```python
from build123d import *

# Parameters (mm, degrees)
SKETCH1_W           = 160
SKETCH1_H           = 50
BOSS_EXTRUDE1_DEPTH = 1.25
SKETCH2_W           = 10
SKETCH2_H           = 2.5
SKETCH2_W_2         = 15
CUT_EXTRUDE1_DEPTH  = 4
SKETCH3_W           = 2.5
SKETCH3_H           = 22.5
CUT_EXTRUDE2_DEPTH  = 84.852549156
CUT_EXTRUDE4_REACH  = 85.853
SKETCH4_R           = 5.5
SKETCH4_R_2         = 2.5


with BuildPart() as part:
    # Sketch1 → Boss-Extrude1 (new, symmetric)
    with BuildSketch(Plane(origin=(0, 0, 0), x_dir=(1, 0, 0), z_dir=(0, 1, 0))):
        Rectangle(SKETCH1_W, SKETCH1_H)
    extrude(amount=BOSS_EXTRUDE1_DEPTH, both=True)

    # Sketch2 → Cut-Extrude1 (cut)
    with BuildSketch(Plane(origin=(0, 1.25, 0), x_dir=(1, 0, 0), z_dir=(0, 1, 0))):
        with Locations((30, 23.75)):
            Rectangle(SKETCH2_W, SKETCH2_H)
        with Locations((10, 23.75)):
            Rectangle(SKETCH2_W, SKETCH2_H)
        with Locations((10, -23.75)):
            Rectangle(SKETCH2_W, SKETCH2_H)
        with Locations((30, -23.75)):
            Rectangle(SKETCH2_W, SKETCH2_H)
        with Locations((50, 23.75)):
            Rectangle(SKETCH2_W, SKETCH2_H)
        with Locations((50, -23.75)):
            Rectangle(SKETCH2_W, SKETCH2_H)
        with Locations((-10, 23.75)):
            Rectangle(SKETCH2_W, SKETCH2_H)
        with Locations((-10, -23.75)):
            Rectangle(SKETCH2_W, SKETCH2_H)
        with Locations((-30, 23.75)):
            Rectangle(SKETCH2_W, SKETCH2_H)
        with Locations((-30, -23.75)):
            Rectangle(SKETCH2_W, SKETCH2_H)
        with Locations((-50, 23.75)):
            Rectangle(SKETCH2_W, SKETCH2_H)
        with Locations((-50, -23.75)):
            Rectangle(SKETCH2_W, SKETCH2_H)
        with Locations((72.5, 23.75)):
            Rectangle(SKETCH2_W_2, SKETCH2_H)
        with Locations((72.5, -23.75)):
            Rectangle(SKETCH2_W_2, SKETCH2_H)
        with Locations((-72.5, 23.75)):
            Rectangle(SKETCH2_W_2, SKETCH2_H)
        with Locations((-72.5, -23.75)):
            Rectangle(SKETCH2_W_2, SKETCH2_H)
    extrude(amount=-CUT_EXTRUDE1_DEPTH, mode=Mode.SUBTRACT)

    # Sketch3 → Cut-Extrude2 (cut, through all)
    with BuildSketch(Plane(origin=(0, 1.25, 0), x_dir=(1, 0, 0), z_dir=(0, 1, 0))):
        with Locations((78.75, -11.25)):
            Rectangle(SKETCH3_W, SKETCH3_H)
        with Locations((-78.75, -11.25)):
            Rectangle(SKETCH3_W, SKETCH3_H)
    extrude(amount=-CUT_EXTRUDE2_DEPTH, mode=Mode.SUBTRACT)

    # Sketch4 → Cut-Extrude4 (cut, up to next)
    with BuildSketch(Plane.XZ.offset(1.25), mode=Mode.PRIVATE) as cut_extrude4_sk1:
        with Locations(Location((-57.7529076, -6.3187203, 0), (0, 0, 270))):
            Circle(SKETCH4_R)
    cut_extrude4_tool1 = extrude(cut_extrude4_sk1.sketch, amount=-CUT_EXTRUDE4_REACH, mode=Mode.PRIVATE) & part.part
    # Sketch4 → Cut-Extrude4 (cut, up to next)
    with BuildSketch(Plane.XZ.offset(1.25), mode=Mode.PRIVATE) as cut_extrude4_sk2:
        with Locations(Location((-27.7529076, 0, 0), (0, 0, 270))):
            Circle(SKETCH4_R_2)
    cut_extrude4_tool2 = extrude(cut_extrude4_sk2.sketch, amount=-CUT_EXTRUDE4_REACH, mode=Mode.PRIVATE) & part.part
    add(cut_extrude4_tool1.solids().sort_by_distance((-57.752908, -1.25, -6.31872))[0], mode=Mode.SUBTRACT)
    add(cut_extrude4_tool2.solids().sort_by_distance((-27.752908, -1.25, 0))[0], mode=Mode.SUBTRACT)


solid = part.part
```
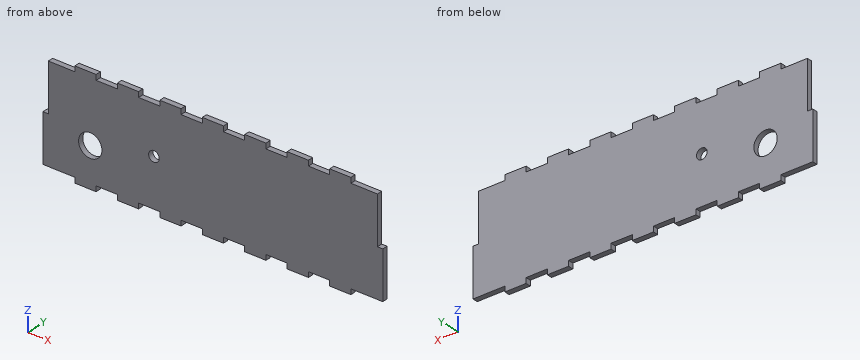
Check sheet for the modelled part. Datum: model origin and axes. Units: mm. Give positions to 0.01 mm unless a question says otherwise; leave off trailing zeros. Order: outer loops, then holes, each group sorted by start corner. A loop starts at its lowest first (then second) coordinate and runs counter-clockwise, first axis right, second up. Notation, with made-up numbers: M -17.75,87.25 L 0.25,87.25 A29 ccw 0.25,114.25 Z; hole C -24,77 d6. An arc over 180 degrees is marked long. Answer in a Markdown table with one row per item. Add a question column.
Q1. Sectioned sample at A-A, the plane z = -6. Record the boundary of the cut face in (x, y), and give its area (3 significant figures).
Q2. Gauge pin test, flat ends, axial feed: pin 1 Ø1.2 at (y, z) = (0, 23.5) entering from +X; pin 2 Ø0.8 at (x, y) = (-8, 0) entering from -Z; pin 3 Ø1 at (y, z) = (-0.5, 17) entering from +X. Record the tip position at first contact, or that the pin passes through.
Q3. Sectioned sample at D-D, the plane y = 0.8. Count the separate pieces of the cut face and the enclosed holes in it, and give its area (3 significant figures).
Q4. Sectioned sample at C-C, the plane z = 7.5. Record the boundary of the cut face in (x, y), and give its area (4 significant figures).
Q5. Sectioned sample at B-B, the plane x = 48. Record the boundary of the cut face in (y, z).
Q6. Thickness scan on L1, parallel to Z at x = 32, y = -0.85; L2, parallel to X at y = 0.05, z = 14; L3, parallel to X at y = 1.15, z = -7.5. Record the ranges inside material, lowest first.
Verdict:
| question | item | result |
|---|---|---|
| 1 | outline | M -80,-1.25 L -63.24,-1.25 L -63.24,1.25 L -80,1.25 Z; M -52.26,-1.25 L 80,-1.25 L 80,1.25 L -52.26,1.25 Z |
| 1 | area | 373 mm² |
| 2 | pin 1 | x = 65 |
| 2 | pin 2 | z = -22.5 |
| 2 | pin 3 | x = 77.5 |
| 3 | separate pieces | 1 |
| 3 | enclosed holes | 2 |
| 3 | area | 7,320 mm² |
| 4 | outline | M -77.5,-1.25 L 77.5,-1.25 L 77.5,1.25 L -77.5,1.25 Z |
| 4 | area | 387.5 mm² |
| 5 | outline | M -1.25,-22.5 L 1.25,-22.5 L 1.25,22.5 L -1.25,22.5 Z |
| 6 | L1 | -22.5 to 22.5 |
| 6 | L2 | -77.5 to 77.5 |
| 6 | L3 | -80 to -63.12, -52.38 to 80 |
